For this review, take the finished solid that the model builds, in its own axes (mm). A direction names the side the tool comes from. Round coordinates to 2 decimals unless told otherwise and drop trailing zeros. Loops run counter-clockwise (first coordinate to the right, second up) from the corner with the lowest first, then second, coordinate; pieces in that order, holes last. Notation, with made-up numbers: (13.5, 6.5) -> (72.5, 6.5) arc R22 cw to (72.5, 20.5) -> close; hole circle Ø7 at (-30, 1). An arc over 180 degrees is marked (long way). One line per question, with ' | ' between items. Start each with the question number.
1. For pin 1 Ø4 at (x, y) = (-1, 81.5) entering from +Z; pin 2 Ø2 at (y, z) = (31.5, -25) entering from +X, all flat-tipped, find the tip position at first contact; note any pin that passes through.
2. Consider section B-B (x = 0). Write out the cut boundary in (y, z) (1 decimal), and give its area (3 significant figures).
3. Wall thickness on line 1 along X through (y, z) = (74, -39) (1 decimal); line 2 along Z through (x, y) = (0, 10.25) (1 decimal); line 3 along Z through (x, y) = (0, 106) (1 decimal): over which ranges is each line inside the solid? List them lowest first.
4. Draft analysis for pull direction X (two halves, no side actions). For faces 1 (the face through (-0.41, 112.99, -51.15)), 2 (the face through (-0.62, 112.21, -52.72)), state which applies: pulls with the +X half, pulls with the -X half, needs draft (parallel to the pull), parting line crosses it, or undercut.
5. For faces 3 (the face through (4.4, 44.49, -26.18)), 4 (the face through (-1.03, 7.43, -3.35)), list the 3-axis set-ups (+Z, -Z, +X, -X, +Y, -Y) from which the entire face can be reached by the end or side of a thin tool; tool diameter is ignored.
```python
from build123d import *

# Parameters (mm, degrees)
SKETCH2_R   = 4.7625
SKETCH2_R_2 = 3.175


with BuildPart() as part:
    # Sweep2: sweep along a path in Sketch4
    with BuildLine(Plane(origin=(0, 0, 0), x_dir=(0, 0, -1), z_dir=(1, 0, 0))) as sweep2_path:
        Line((8, 0), (8, 14))
        Line((8, 14), (28, 14))
        Line((28, 14), (28, 74))
        Line((28, 74), (48, 74))
        Line((48, 74), (48, 154))
    # Sketch2 → Sweep2 (sweep)
    with BuildSketch(Plane(origin=(0, 0, 0), x_dir=(1, 0, 0), z_dir=(0, 1, 0))):
        with Locations((0, 8)):
            Circle(SKETCH2_R)
        with Locations((0, 8)):
            Circle(SKETCH2_R_2, mode=Mode.SUBTRACT)
    sweep(path=sweep2_path.line, transition=Transition.RIGHT)


solid = part.part
```
Answer block:
1) pin 1: stops at z = -43.24 | pin 2: stops at x = 4.32
2) outline: (0, -12.8) -> (9.2, -12.8) -> (9.2, -32.8) -> (69.2, -32.8) -> (69.2, -52.8) -> (154, -52.8) -> (154, -51.2) -> (70.8, -51.2) -> (70.8, -31.2) -> (10.8, -31.2) -> (10.8, -11.2) -> (0, -11.2) -> close; (0, -4.8) -> (17.2, -4.8) -> (17.2, -24.8) -> (77.2, -24.8) -> (77.2, -44.8) -> (154, -44.8) -> (154, -43.2) -> (78.8, -43.2) -> (78.8, -23.2) -> (18.8, -23.2) -> (18.8, -3.2) -> (0, -3.2) -> close | area: 616 mm2
3) line 1: x = -4.8 to -3.2, 3.2 to 4.8 | line 2: z = -32.8 to -11.2, -4.8 to -3.2 | line 3: z = -52.8 to -51.2, -44.8 to -43.2
4) face 1: undercut | face 2: parting line crosses it
5) face 3: none | face 4: -Y
